Part print with two shaded views. Sizes in mm from the minimum x, y, z corner. A direction names the side the tool comes from. Round coordinates to 2 decimals unless told otherwise and drop trailing zeros. Loops run counter-clockwise (first coordinate to the right, second up) from the corner with the lowest first, then second, coordinate; pieces in that order, holes last.
(1) Cut at A-A on z = 4. List the corners of the cut face in (x, y).
(2) Flat gauge pins, fed straight in: pin 1 (0.5 mm diameter, centred on y = 0.5, z = 9, fed in from -X); pin 2 (1.8 mm diameter, centred on x = 6.44, y = 3, fed in from +Z). Where does each tip first touch, or does it go through?
(3) Tool access for the marked faces 4, 5, 6 and 7: list every direction of +Z, -Z, +X, -X, +Y, -Y with a clear straight run to the whole face (end or side of a thin tool).
(4) Cut at D-D on z = 8.25. List the corners of the cut face in (x, y).
(5) Cut at B-B on y = 3. List the corners of the cut face in (x, z), then the cut area to 3 significant figures.
(6) Cut at C-C on x = 6.44. List the corners of the cut face in (y, z).
(7) Mould opens along Z. For the marked faces 1, 2 and 3 say: +Z half, -Z half, draft (parallel to the pull), parting line (faces both ways), or undercut.
(8) Probe probe 1 along Z at (x, y) = (13.25, 2.95); probe 2 along X at (y, z) = (5, 5.5); probe 3 along Y at (x, z) = (15.56, 8.15). List the from-to ranges inside material, lowest first.
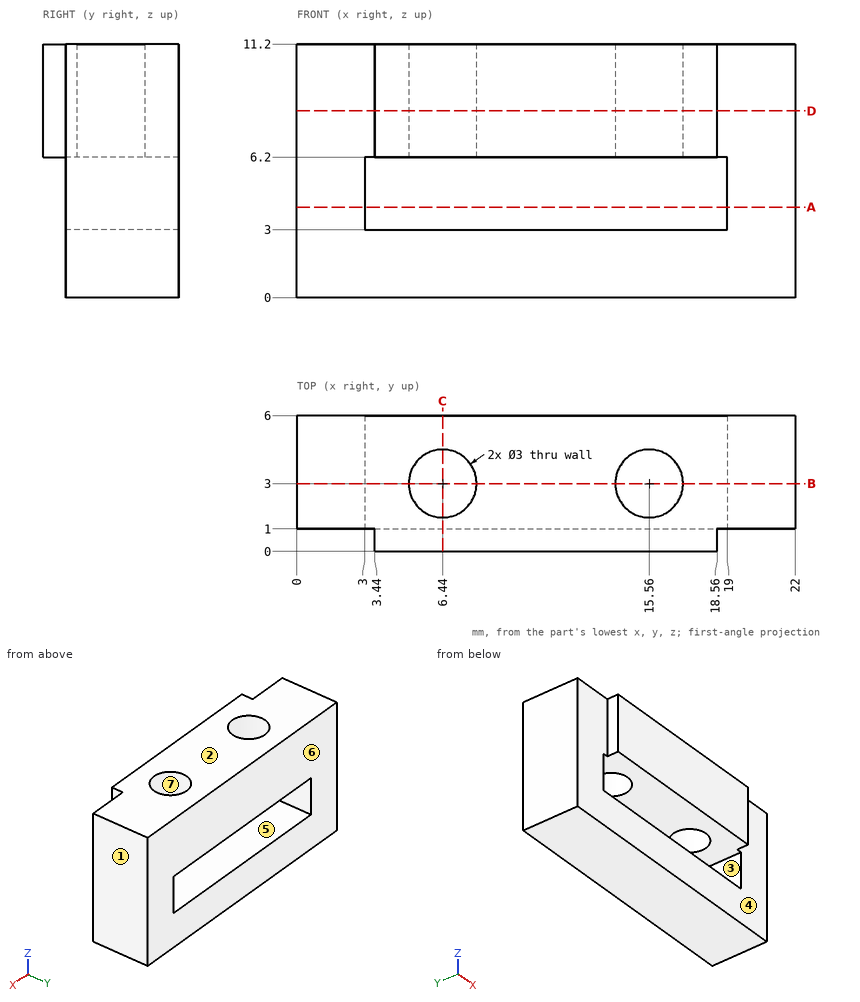
Final values:
1. outline: (0, 1) - (3, 1) - (3, 6) - (0, 6) - close; (19, 1) - (22, 1) - (22, 6) - (19, 6) - close
2. pin 1: stops at x = 3.44
2. pin 2: stops at z = 3
3. face 4: -Z, -Y
3. face 5: +Y, -Y
3. face 6: +Z, -Z, +X, -X, +Y
3. face 7: +Z
4. outline: (0, 1) - (3.44, 1) - (3.44, 0) - (18.56, 0) - (18.56, 1) - (22, 1) - (22, 6) - (0, 6) - close; hole circle Ø3 at (6.44, 3); hole circle Ø3 at (15.56, 3)
5. outline: (0, 0) - (22, 0) - (22, 11.2) - (17.06, 11.2) - (17.06, 6.2) - (19, 6.2) - (19, 3) - (3, 3) - (3, 6.2) - (4.94, 6.2) - (4.94, 11.2) - (0, 11.2) - close; (7.94, 6.2) - (14.06, 6.2) - (14.06, 11.2) - (7.94, 11.2) - close
5. area: 165 mm2
6. outline: (0, 6.2) - (1.5, 6.2) - (1.5, 11.2) - (0, 11.2) - close; (1, 0) - (6, 0) - (6, 3) - (1, 3) - close; (4.5, 6.2) - (6, 6.2) - (6, 11.2) - (4.5, 11.2) - close
7. face 1: draft
7. face 2: +Z half
7. face 3: undercut
8. probe 1: z = 0 to 3, 6.2 to 11.2
8. probe 2: x = 0 to 3, 19 to 22
8. probe 3: y = 0 to 1.5, 4.5 to 6
